The listing builds one solid part. Answer for the finished solid, in the listing's coordinates (mm). A direction names the side the tool comes from. Coordinates: 2 decimals unless noted, no trailing zeros. Write each loop counter-clockwise with the first axis right and the second up, starting at its lowest first coordinate (ties: lowest second). Pieces come first, ordered by that corner, then holes.
```python
from build123d import *

# Parameters (mm, degrees)
SKETCH1_R           = 1.5
BOSS_EXTRUDE1_DEPTH = 3.75
FILLET1_R           = 1.875
CUT_EXTRUDE1_DEPTH  = 2.75
FILLET2_R           = 3


with BuildPart() as part:
    # Sketch1 → Boss-Extrude1 (new body)
    with BuildSketch(Plane(origin=(0, 0, 0), x_dir=(1, 0, 0), z_dir=(0, 1, 0))):
        Polygon((0, 0), (37.5, 0), (37.5, 48), (29.5, 48), (29.5, 50), (8, 50), (8, 48), (0, 48), align=None)
        with Locations(Location((5, 45, 0), (0, 0, 270))):
            Circle(SKETCH1_R, mode=Mode.SUBTRACT)
        with Locations(Location((32.5, 45, 0), (0, 0, 270))):
            Circle(SKETCH1_R, mode=Mode.SUBTRACT)
    extrude(amount=BOSS_EXTRUDE1_DEPTH)

    # Fillet1
    fillet1_edges = [part.edges().sort_by_distance(p)[0] for p in [
        (18.75, 0, 0),
        (18.75, 3.75, 0),
    ]]
    fillet(fillet1_edges, radius=FILLET1_R - 0.0001)  # a hair under: the kernel refuses the full size

    # Sketch2 → Cut-Extrude1 (cut)
    with BuildSketch(Plane(origin=(0, 3.75, 0), x_dir=(1, 0, 0), z_dir=(0, 1, 0))):
        with BuildLine():
            Line((8, 48), (0, 48))
            Line((0, 48), (0, 42))
            Line((0, 42), (5, 42))
            ThreePointArc((5, 42), (7.121320344, 42.878679656), (8, 45))
            Line((8, 45), (8, 48))
        make_face()
        with BuildLine():
            Line((29.5, 48), (37.5, 48))
            Line((37.5, 48), (37.5, 42))
            Line((37.5, 42), (32.5, 42))
            ThreePointArc((32.5, 42), (30.378679656, 42.878679656), (29.5, 45))
            Line((29.5, 45), (29.5, 48))
        make_face()
    extrude(amount=-CUT_EXTRUDE1_DEPTH, mode=Mode.SUBTRACT)

    # Fillet2
    fillet2_edges = [part.edges().sort_by_distance(p)[0] for p in [
        (0, 0.5, -48),
        (37.5, 0.5, -48),
    ]]
    fillet(fillet2_edges, radius=FILLET2_R)


solid = part.part
```
(1) Which of the six approach directions +Z, -Z, +X, -X, +Y, -Y give full straight-line access (tool end or side, diameter ignored) to faces 1 (the flat face through (35, 2, -42)), 2 (the flat face through (32, 0.5, -48)), 3 (the flat face through (2, 2, -42)), 4 (the flat face through (18, 0, -26))?
(2) For a pull along Z with two mould halves and no side action, classify faces 5 (the cylindrical face through (31.6, 0.5, -46.2)), 6 (the cylindrical face through (19, 0.6, -0.5)), 7 (the flat face through (34.4, 1, -45)) as pulls with the +Z half, pulls with the -Z half, needs draft (parallel to the pull), parting line crosses it, or undercut.
(3) Section A-A, the plane y = 2.95 is taken. Write down the section's boundary in (x, z), plus the area to 3 significant figures.
(4) Find the intervals of material crossed by probe 1 along X at (y, z) = (0.85, -45); probe 2 along Z at (x, y) = (5, 0.4); probe 3 along Z at (x, y) = (32.5, 0.55), in increasing order.
(5) Each of these flat-tipped pins is pushed along its axis until it touches: pin 1 (1.1 mm diameter, centred on y = 1.5, z = -48.5, fed in from -X); pin 2 (5 mm diameter, centred on x = 3, z = -45, fed in from +Y); pin 3 (0.8 mm diameter, centred on x = 6.5, y = 0.5, fed in from -Z). Where does it stop, or does it pass through?
Solution:
1. face 1: -Z, +X, +Y
1. face 2: -Z, +X, +Y, -Y
1. face 3: -Z, -X, +Y
1. face 4: +Z, -Z, +X, -X, -Y
2. face 5: undercut
2. face 6: pulls with the +Z half
2. face 7: needs draft
3. outline: (0, -42) - (5, -42) arc R3 cw to (8, -45) - (8, -50) - (29.5, -50) - (29.5, -45) arc R3 cw to (32.5, -42) - (37.5, -42) - (37.5, -0.34) - (0, -0.34) - close
3. area: 1,740 mm2
4. probe 1: x = 0 to 3.5, 6.5 to 31, 34 to 37.5
4. probe 2: z = -48 to -46.5, -43.5 to -0.72
4. probe 3: z = -48 to -46.5, -43.5 to -0.55
5. pin 1: stops at x = 8
5. pin 2: stops at y = 1
5. pin 3: stops at z = -48
